from build123d import *

# Parameters (mm, degrees)
SKETCH1_R               = 12.7
SKETCH1_R_2             = 6.35
BOSS_EXTRUDE1_DEPTH     = 203.2
SKETCH1_3_R             = 6.35
BOSS_EXTRUDE2_DEPTH     = 25.4
SKETCH3_R               = 3.96875
CUT_EXTRUDE2_DEPTH      = 204.992205733
CUT_EXTRUDE2_DEPTH_BACK = 204.992205733


with BuildPart() as part:
    # Sketch1 → Boss-Extrude1 (new body)
    with BuildSketch(Plane(origin=(0, 0, 0), x_dir=(1, 0, 0), z_dir=(0, 1, 0))):
        with Locations(Location((0, 0, 0), (0, 0, 270))):
            Circle(SKETCH1_R)
        Circle(SKETCH1_R_2, mode=Mode.SUBTRACT)
        Circle(SKETCH1_R_2)
    extrude(amount=BOSS_EXTRUDE1_DEPTH)

    # Sketch1_3 → Boss-Extrude2 (add)
    with BuildSketch(Plane(origin=(0, 0, 0), x_dir=(1, 0, 0), z_dir=(0, 1, 0))):
        with Locations(Location((0, 0, 0), (0, 0, 270))):
            Circle(SKETCH1_3_R)
    extrude(amount=-BOSS_EXTRUDE2_DEPTH)

    # Sketch3 → Cut-Extrude2 (cut, two sides)
    with BuildSketch(Plane.XY) as cut_extrude2_sk:
        with Locations((0, -15.875)):
            Circle(SKETCH3_R)
    extrude(amount=CUT_EXTRUDE2_DEPTH, mode=Mode.SUBTRACT)
    extrude(cut_extrude2_sk.sketch, amount=-CUT_EXTRUDE2_DEPTH_BACK, mode=Mode.SUBTRACT)


solid = part.part
Read the model definition and answer for the solid it produces. Units are mm, in the model's axes. A direction names the side the tool comes from. Give positions to 0.01 mm unless a question says otherwise; leave off trailing zeros. Write each loop counter-clockwise with the first axis right and the second up, starting at its lowest first coordinate (ties: lowest second). Pieces come first, ordered by that corner, then holes. Notation, with made-up numbers: (-5.75, -9.5) - (46.25, -9.5) arc R10 ccw to (46.25, 2.5) - close; hole circle Ø4 at (-33.5, -38). An arc over 180 degrees is marked (long way). Use CSV: the item, a comma, the result in double quotes. Start each with the question number.
Item 1: The part is cut by section D-D, the plane x = -9.25. Give the vertices of the cut face in (y, z).
Item 2: The part is cut by section C-C, the plane y = -8.5. Give the vertices of the cut face in (x, z), and give its area (3 significant figures).
Item 3: The part is cut by section B-B, the plane z = -2.5. Give the vertices of the cut face in (x, y) (1 decimal), and give its area (3 significant figures).
Item 4: For faces 1 (the flat face through (0, -25.4, 0)), 2 (the flat face through (6, 0, 3)), determine the directions among +Z, -Z, +X, -X, +Y, -Y from which every point of the face is accessible in a straight line to the end or side of a thin tool.
Item 5: The part is cut by section A-A, the plane x = 0. Give the vertices of the cut face in (y, z).
Item 6: Flat-ended cylindrical pins translate along their axes: P1, Ø1, axis at y = 143.5, z = -4, coming from the -X side; P2, Ø10.5, axis at x = 0, y = -15.875, coming from the +Z side; P3, Ø2, axis at x = 7, z = -6, coming from the -Y side. Find the tip coordinate at first contact, or state that the pin passes through.
Item 7: Consider line 1 (Y direction, x = 0, z = -4.75); line 2 (Z direction, x = 11, y = 66); line 3 (Y direction, x = 7, z = -10). Determine where each line is inside the solid, lowest interval first.
Taken from the geometry:
1,outline,"(0, -8.7) - (203.2, -8.7) - (203.2, 8.7) - (0, 8.7) - close"
2,outline,"circle Ø12.7 at (0, 0)"
2,area,"127 mm2"
3,outline,"(-12.5, 0) - (-5.8, 0) - (-5.8, -25.4) - (5.8, -25.4) - (5.8, 0) - (12.5, 0) - (12.5, 203.2) - (-12.5, 203.2) - close; hole circle Ø7.9 at (0, -15.9)"
3,area,"5,310 mm2"
4,face 1,"+Z, -Z, +X, -X, -Y"
4,face 2,"-Y"
5,outline,"(-25.4, -6.35) - (-19.84, -6.35) - (-19.84, 6.35) - (-25.4, 6.35) - close; (-11.91, -6.35) - (0, -6.35) - (0, -12.7) - (203.2, -12.7) - (203.2, 12.7) - (0, 12.7) - (0, 6.35) - (-11.91, 6.35) - close"
6,P1,"x = -12.21"
6,P2,"z = 6.35"
6,P3,"y = 0"
7,line 1,"-25.4 to -19.84, -11.91 to 203.2"
7,line 2,"-6.35 to 6.35"
7,line 3,"0 to 203.2"
